```python
from build123d import *

# Parameters (mm, degrees)
SKETCH_1_W          = 150
SKETCH_1_H          = 50
EXTRUDE_1_DEPTH     = 10
CUT_EXTRUDE_1_DEPTH = 150
SKETCH_3_W          = 20.4
SKETCH_3_H          = 1
CUT_EXTRUDE_2_DEPTH = 150
SKETCH_4_W          = 20.4
SKETCH_4_H          = 5
EXTRUDE_2_DEPTH     = 12
SKETCH_5_R          = 3.01
EXTRUDE_3_DEPTH     = 45
CHAMFER_2_SIZE      = 1


with BuildPart() as part:
    # 草图1 → 凸台-拉伸1 (new body)
    with BuildSketch(Plane.XY):
        with Locations((50.269431659, 25)):
            Rectangle(SKETCH_1_W, SKETCH_1_H)
    extrude(amount=EXTRUDE_1_DEPTH)

    # 草图2 → 切除-拉伸1 (cut)
    with BuildSketch(Plane(origin=(125.269431659, 0, 0), x_dir=(0, 0, -1), z_dir=(1, 0, 0))):
        Polygon((-3, 13), (-3, 37), (-5.2, 37), (-5.2, 33), (-10, 33), (-10, 17), (-5.2, 17), (-5.2, 13), align=None)
    extrude(amount=-CUT_EXTRUDE_1_DEPTH, mode=Mode.SUBTRACT)

    # 草图3 → 切除-拉伸2 (cut)
    with BuildSketch(Plane(origin=(0, 50, 0), x_dir=(1, 0, 0), z_dir=(0, 1, 0))):
        with Locations((50.269431659, -0.5)):
            Rectangle(SKETCH_3_W, SKETCH_3_H)
    extrude(amount=-CUT_EXTRUDE_2_DEPTH, mode=Mode.SUBTRACT)

    # 草图4 → 凸台-拉伸2 (add)
    with BuildSketch(Plane(origin=(0, 0, 1), x_dir=(-1, 0, 0), z_dir=(0, 0, -1))):
        with Locations((-50.269431659, 2.5)):
            Rectangle(SKETCH_4_W, SKETCH_4_H)
    extrude(amount=EXTRUDE_2_DEPTH)

    # 草图5 → 凸台-拉伸3 (add)
    with BuildSketch(Plane(origin=(0, 5, 0), x_dir=(1, 0, 0), z_dir=(0, 1, 0))):
        with Locations((50.269431659, 8)):
            Circle(SKETCH_5_R)
    extrude(amount=EXTRUDE_3_DEPTH)

    # 倒角2
    chamfer_2_edges = [part.edges().sort_by_distance(p)[0] for p in [
        (47.259431659, 50, -8),
    ]]
    chamfer(chamfer_2_edges, length=CHAMFER_2_SIZE)


solid = part.part
```
CAD build for the part. Positions are in the model's coordinates, mm. A direction names the side the tool comes from. Give positions to 0.01 mm unless a question says otherwise; leave off trailing zeros. Loops run counter-clockwise (first coordinate to the right, second up) from the corner with the lowest first, then second, coordinate; pieces in that order, holes last. Notation, with made-up numbers: (70.5, -35.75) - (129.5, -35.75) arc R17 ccw to (129.5, -11.75) - close; hole circle Ø3 at (-16.75, -16). An arc over 180 degrees is marked (long way). Put each result on its own line as item: value.
Q1. Probe line 1 along X through (y, z) = (41, 0.5); line 2 along Z through (x, y) = (96.5, 15); line 3 along Y through (x, z) = (116, 3.25). List the from-to ranges inside material, lowest first.
Filled in:
line 1: x = -24.73 to 40.07, 60.47 to 125.27
line 2: z = 0 to 3, 5.2 to 10
line 3: y = 0 to 13, 37 to 50
Q2. Slice it at D-D (z = -8). Give the cut face in (x, y).
Filled in:
outline: (40.07, 0) - (60.47, 0) - (60.47, 5) - (53.28, 5) - (53.28, 49) - (52.28, 50) - (48.26, 50) - (47.26, 49) - (47.26, 5) - (40.07, 5) - close
Q3. Slice it at B-B (z = 8.5). Give the cut face in (x, y).
Filled in:
outline: (-24.73, 0) - (125.27, 0) - (125.27, 17) - (-24.73, 17) - close; (-24.73, 33) - (125.27, 33) - (125.27, 50) - (-24.73, 50) - close
Q4. Slice it at C-C (x = 75). Give the cut face in (y, z).
Filled in:
outline: (0, 0) - (50, 0) - (50, 10) - (33, 10) - (33, 5.2) - (37, 5.2) - (37, 3) - (13, 3) - (13, 5.2) - (17, 5.2) - (17, 10) - (0, 10) - close
Q5. Tool access for faces 4 (the face through (40.069, 2, -5)), 5 (the face through (50, 28, 1)), 6 (the face through (60.469, 2, -5)): list every direction of +Z, -Z, +X, -X, +Y, -Y with a clear straight run to the whole face (end or side of a thin tool).
Filled in:
face 4: -Z, -X, +Y, -Y
face 5: +Y
face 6: -Z, +X, +Y, -Y
Q6. Mould opens along Y. For faces 1 (the face through (125.269, 24.7, 2.7)), 2 (the face through (51, 0, 4)), 3 (the face through (51, 17, 8)) say: pulls with the +Y half, pulls with the -Y half, needs draft (parallel to the pull), parting line crosses it, or undercut.
Filled in:
face 1: needs draft
face 2: pulls with the -Y half
face 3: undercut
Q7. Flat gauge pins, fed straight in: pin 1 (1 mm diameter, centred on y = 20.5, z = -5.5, fed in from -X); pin 2 (1.5 mm diameter, centred on x = 64.5, y = 27.5, fed in from -Z); pin 3 (5.5 mm diameter, centred on y = 2, z = -4.5, fed in from +X); pin 4 (1.1 mm diameter, centred on x = 31.5, z = 4.5, fed in from -Y). Where does each tip first touch, or does it go through?
Filled in:
pin 1: stops at x = 48.02
pin 2: stops at z = 0
pin 3: stops at x = 60.47
pin 4: stops at y = 0
Q8. Slice it at A-A (y = 21). Give the cut face in (x, z), plus the area to 3 significant figures.
Filled in:
outline: (-24.73, 0) - (40.07, 0) - (40.07, 1) - (60.47, 1) - (60.47, 0) - (125.27, 0) - (125.27, 3) - (-24.73, 3) - close; circle Ø6.02 at (50.27, -8)
area: 458 mm²
